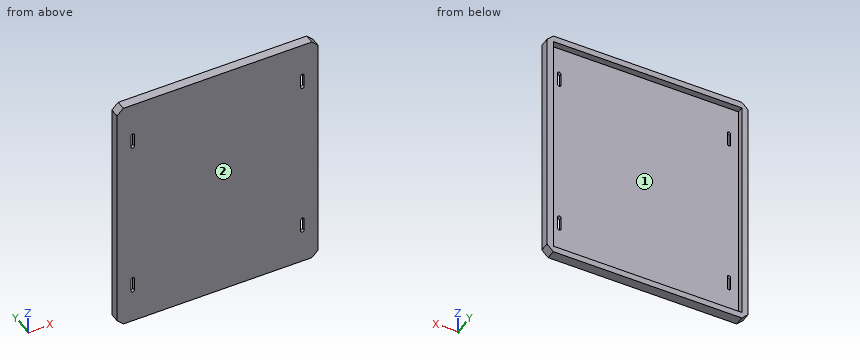
```python
from build123d import *

# Parameters (mm, degrees)
SKETCH_1_W          = 320
SKETCH_1_H          = 390
EXTRUDE_1_DEPTH     = 5
CUT_EXTRUDE_1_DEPTH = 5
SKETCH_3_W          = 320
SKETCH_3_H          = 390
SKETCH_3_W_2        = 300
SKETCH_3_H_2        = 370
EXTRUDE_2_DEPTH     = 15
CHAMFER_1_SIZE      = 10


with BuildPart() as part:
    # 草图1 → 凸台-拉伸1 (new body)
    with BuildSketch(Plane(origin=(0, 0, 0), x_dir=(1, 0, 0), z_dir=(0, 1, 0))):
        Rectangle(SKETCH_1_W, SKETCH_1_H)
    extrude(amount=EXTRUDE_1_DEPTH)

    # 草图2 → 切除-拉伸1 (cut)
    with BuildSketch(Plane(origin=(0, 5, 0), x_dir=(1, 0, 0), z_dir=(0, 1, 0))):
        with BuildLine():
            Line((-132.25, 140), (-132.25, 120))
            ThreePointArc((-132.25, 120), (-135, 117.25), (-137.75, 120))
            Line((-137.75, 120), (-137.75, 140))
            ThreePointArc((-137.75, 140), (-135, 142.75), (-132.25, 140))
        make_face()
        with BuildLine():
            Line((-132.25, -140), (-132.25, -120))
            ThreePointArc((-132.25, -120), (-135, -117.25), (-137.75, -120))
            Line((-137.75, -120), (-137.75, -140))
            ThreePointArc((-137.75, -140), (-135, -142.75), (-132.25, -140))
        make_face()
        with BuildLine():
            Line((132.25, 140), (132.25, 120))
            ThreePointArc((132.25, 120), (135, 117.25), (137.75, 120))
            Line((137.75, 120), (137.75, 140))
            ThreePointArc((137.75, 140), (135, 142.75), (132.25, 140))
        make_face()
        with BuildLine():
            Line((132.25, -140), (132.25, -120))
            ThreePointArc((132.25, -120), (135, -117.25), (137.75, -120))
            Line((137.75, -120), (137.75, -140))
            ThreePointArc((137.75, -140), (135, -142.75), (132.25, -140))
        make_face()
    extrude(amount=-CUT_EXTRUDE_1_DEPTH, mode=Mode.SUBTRACT)

    # 草图3 → 凸台-拉伸2 (add)
    with BuildSketch(Plane(origin=(0, 0, 0), x_dir=(1, 0, 0), z_dir=(0, 1, 0))):
        Rectangle(SKETCH_3_W, SKETCH_3_H)
        Rectangle(SKETCH_3_W_2, SKETCH_3_H_2, mode=Mode.SUBTRACT)
    extrude(amount=EXTRUDE_2_DEPTH)

    # 倒角1
    chamfer_1_edges = [part.edges().sort_by_distance(p)[0] for p in [
        (-160, 7.5, -195),
        (-160, 7.5, 195),
        (160, 7.5, 195),
        (160, 7.5, -195),
    ]]
    chamfer(chamfer_1_edges, length=CHAMFER_1_SIZE)


solid = part.part
```
Can you work these out from the model? Positions are in its coordinate system, mm. Face numbers are marked on the shaded views. Round coordinates to 2 decimals unless told otherwise and drop trailing zeros. Loops run counter-clockwise (first coordinate to the right, second up) from the corner with the lowest first, then second, coordinate; pieces in that order, holes last. Notation, with made-up numbers: (-3.75, 48) -> (16.25, 48) arc R34 cw to (16.25, 84) -> close; hole circle Ø8 at (-37, 35). An arc over 180 degrees is marked (long way). Answer in a Markdown table with one row per item.
Item 1: Suppose I cut it at A-A, the plane y = 9.5. List the corners of the cut face in (x, z) for me.
Answer block:
| item | result |
|---|---|
| outline | (-160, -185) -> (-150, -195) -> (150, -195) -> (160, -185) -> (160, 185) -> (150, 195) -> (-150, 195) -> (-160, 185) -> close; hole (-150, -185) -> (150, -185) -> (150, 185) -> (-150, 185) -> close |
Item 2: Will this pin go through, and if not, where does the flat tip stop? P1, Ø3, axis at x = -37.5, z = -16.5, coming from the +Y side.
Answer block:
| item | result |
|---|---|
| P1 | y = 5 |
Item 3: Suppose I cut it at C-C, the plane z = 67.5. List the corners of the cut face in (x, y) for me, plus the area to 3 significant figures.
Answer block:
| item | result |
|---|---|
| outline | (-160, 0) -> (160, 0) -> (160, 15) -> (150, 15) -> (150, 5) -> (-150, 5) -> (-150, 15) -> (-160, 15) -> close |
| area | 1,800 mm² |
Item 4: Suppose I cut it at B-B, the plane x = 4.5. List the corners of the cut face in (y, z) for me, plus the area to 3 significant figures.
Answer block:
| item | result |
|---|---|
| outline | (0, -195) -> (15, -195) -> (15, -185) -> (5, -185) -> (5, 185) -> (15, 185) -> (15, 195) -> (0, 195) -> close |
| area | 2,150 mm² |
Item 5: If I drill on probe 1 along X at (y, z) = (7, 140); probe 2 along Z at (x, y) = (-17.5, 6.75); probe 3 along Y at (x, z) = (116, -60), over which ranges is the centre line in solid material (lowest first)?
Answer block:
| item | result |
|---|---|
| probe 1 | -160 to -150, 150 to 160 |
| probe 2 | -195 to -185, 185 to 195 |
| probe 3 | 0 to 5 |
Item 6: We'd pull the mould along X, two halves only. Please class the marked faces 1 and 2: released by +X, released by -X, zero draft, split by the parting line, or undercut.
Answer block:
| item | result |
|---|---|
| face 1 | undercut |
| face 2 | zero draft |
